Geometry: final body of the model. Coordinates: model frame, mm. Give positions to 0.01 mm unless a question says otherwise; leave off trailing zeros. Loops run counter-clockwise (first coordinate to the right, second up) from the corner with the lowest first, then second, coordinate; pieces in that order, holes last. Notation, with made-up numbers: (54.5, 81.5) - (69.5, 81.5) arc R25 cw to (69.5, 108.5) - close; hole circle Ø7 at (3.25, 70.5). An arc over 180 degrees is marked (long way). Answer in a Markdown table with one row per item.
from build123d import *


with BuildPart() as part:
    # Sketch1 → Revolve1 (revolve)
    with BuildSketch(Plane(origin=(0, 0, 0), x_dir=(0, 0, -1), z_dir=(1, 0, 0))):
        with BuildLine():
            Line((-2.5, 7), (-2.5, 7.8))
            ThreePointArc((-2.5, 7.8), (-2.441421356, 7.941421356), (-2.3, 8))
            Line((-2.3, 8), (2.3, 8))
            ThreePointArc((2.3, 8), (2.441421356, 7.941421356), (2.5, 7.8))
            Line((2.5, 7.8), (2.5, 7))
            Line((2.5, 7), (2.2, 7))
            Line((2.2, 7), (2.2, 6.7))
            Line((2.2, 6.7), (2.1, 6.7))
            Line((2.1, 6.7), (2.4, 6.4))
            Line((2.4, 6.4), (2.4, 5.202907901))
            Line((2.4, 5.202907901), (2.3, 5.202907901))
            Line((2.3, 5.202907901), (2.3, 6.358578644))
            Line((2.3, 6.358578644), (1.958578644, 6.7))
            Line((1.958578644, 6.7), (0.714142843, 6.7))
            ThreePointArc((0.714142843, 6.7), (0, 7), (-0.714142843, 6.7))
            Line((-0.714142843, 6.7), (-1.958578644, 6.7))
            Line((-1.958578644, 6.7), (-2.3, 6.358578644))
            Line((-2.3, 6.358578644), (-2.3, 5.202907901))
            Line((-2.3, 5.202907901), (-2.4, 5.202907901))
            Line((-2.4, 5.202907901), (-2.4, 6.4))
            Line((-2.4, 6.4), (-2.1, 6.7))
            Line((-2.1, 6.7), (-2.2, 6.7))
            Line((-2.2, 6.7), (-2.2, 7))
            Line((-2.2, 7), (-2.5, 7))
        make_face()
    revolve(axis=Axis((0, 0, 6.755399071), (0, 0, -1)))


solid = part.part
Q1. Cut plane B-B (z = 0). Output: boundary loops of the cut face in (x, y).
Check values:
| item | result |
|---|---|
| outline | circle Ø16 at (0, 0); hole circle Ø14 at (0, 0) |
Q2. Material intervals for line 1 along X through (y, z) = (0, 0.85); line 2 along X through (y, z) = (0, 2.35); line 3 along X through (y, z) = (2.5, -0.2), sorted ascending.
Check values:
| item | result |
|---|---|
| line 1 | -8 to -6.7, 6.7 to 8 |
| line 2 | -7.99 to -7, -6.45 to -5.2, 5.2 to 6.45, 7 to 7.99 |
| line 3 | -7.6 to -6.52, 6.52 to 7.6 |
Q3. Draft query along Z for faces 1 (the flat face through (4, 6, 2.5)), 2 (the cylindrical face through (-7.81, -1.73, -0.03)), 3 (the cylindrical face through (0.295, -6.694, -1.328)). Return one class per face: pulls with the +Z half, pulls with the -Z half, needs draft (parallel to the pull), parting line crosses it, or undercut.
Check values:
| item | result |
|---|---|
| face 1 | pulls with the +Z half |
| face 2 | needs draft |
| face 3 | undercut |
Q4. Cut plane A-A (z = -1.6). Output: boundary loops of the cut face in (x, y), and give its area (3 significant figures).
Check values:
| item | result |
|---|---|
| outline | circle Ø16 at (0, 0); hole circle Ø13.4 at (0, 0) |
| area | 60.0 mm² |
Q5. First-contact query: pin 1 (8 mm diameter, centred on x = 0, y = 0, fed in from -Z); pin 2 (6 mm diameter, centred on x = -0.5, y = -3.5, fed in from +Z); pin 3 (2 mm diameter, centred on x = 2, z = 1.5, fed in from +Y); pin 4 (2 mm diameter, centred on y = -2, z = -0.5, fed in from -X). Flat tips, straight axial feed; report the tip coordinate or a pass-through.
Check values:
| item | result |
|---|---|
| pin 1 | through |
| pin 2 | z = 2.4 |
| pin 3 | y = 7.94 |
| pin 4 | x = -7.94 |
